from build123d import *

# Parameters (mm, degrees)
SKETCH_1_W          = 100
SKETCH_1_H          = 100
EXTRUDE_1_DEPTH     = 25
SKETCH_2_W          = 100
SKETCH_2_H          = 100
SKETCH_2_W_2        = 8
SKETCH_2_H_2        = 8
CUT_EXTRUDE_1_DEPTH = 20
EXTRUDE_2_REACH     = 145.614
SKETCH_3_R          = 5


with BuildPart() as part:
    # 草图1 → 凸台-拉伸1 (new body)
    with BuildSketch(Plane.XY):
        with Locations((50, 50)):
            Rectangle(SKETCH_1_W, SKETCH_1_H)
    extrude(amount=EXTRUDE_1_DEPTH)

    # 草图2 → 切除-拉伸1 (cut)
    with BuildSketch(Plane.XY.offset(25)):
        with Locations((50, 50)):
            Rectangle(SKETCH_2_W, SKETCH_2_H)
        with Locations((14, 86)):
            Rectangle(SKETCH_2_W_2, SKETCH_2_H_2, mode=Mode.SUBTRACT)
        with Locations((86, 86)):
            Rectangle(SKETCH_2_W_2, SKETCH_2_H_2, mode=Mode.SUBTRACT)
        with Locations((14, 14)):
            Rectangle(SKETCH_2_W_2, SKETCH_2_H_2, mode=Mode.SUBTRACT)
        with Locations((86, 14)):
            Rectangle(SKETCH_2_W_2, SKETCH_2_H_2, mode=Mode.SUBTRACT)
    extrude(amount=-CUT_EXTRUDE_1_DEPTH, mode=Mode.SUBTRACT)

    # 草图3 → 凸台-拉伸2 (add, up to next)
    with BuildSketch(Plane.XY.offset(25), mode=Mode.PRIVATE) as extrude_2_sk1:
        with Locations((50, 50)):
            Circle(SKETCH_3_R)
    extrude_2_tool1 = extrude(extrude_2_sk1.sketch, amount=-EXTRUDE_2_REACH, mode=Mode.PRIVATE) - part.part
    add(extrude_2_tool1.solids().sort_by_distance((50, 50, 25))[0])


solid = part.part
Geometry: final body of the model. Coordinates: model frame, mm. A direction names the side the tool comes from. Give positions to 0.01 mm unless a question says otherwise; leave off trailing zeros. Loops run counter-clockwise (first coordinate to the right, second up) from the corner with the lowest first, then second, coordinate; pieces in that order, holes last. Notation, with made-up numbers: (10, -30) - (61, -30) arc R25 ccw to (61, -12) - close; hole circle Ø4 at (20, 33.5). An arc over 180 degrees is marked (long way). One line per question, with ' | ' between items. Start each with the question number.
(1) Section query B-B on y = 50. Return loops of the section in (x, z), then the cut area to 3 significant figures.
(2) Pull-direction query (X, two-part tool) for faces 1 (the flat face through (82, 14, 15)), 2 (the flat face through (86, 90, 15)), 3 (the flat face through (0, 49, 2)); classes: released by +X, released by -X, zero draft, split by the parting line, or undercut.
(3) Reachability of faces 4 (the flat face through (90, 14, 15)), 5 (the flat face through (10, 86, 15)), 6 (the flat face through (18, 86, 15)), 7 (the flat face through (14, 10, 15)), 8 (the flat face through (86, 18, 15)) from +Z, -Z, +X, -X, +Y, -Y: full face, straight path, thin tool, end or side. Return the list, or none.
(4) Section query A-A on z = 9.5. Return loops of the section in (x, y).
(5) Contact query for flat-ended pins moving along their axis: pin 1 (4 mm diameter, centred on x = 87, z = 11, fed in from +Y); pin 2 (2.5 mm diameter, centred on y = 12.5, z = 20, fed in from -X); pin 3 (6.5 mm diameter, centred on x = 12.5, z = 18.5, fed in from -Y). Output: stop coordinate, or through.
(6) Section query C-C on x = 16. Return loops of the section in (y, z).
(7) Ray query, line 1 (X direction, y = 89, z = 9.5); line 2 (Z direction, x = 60, y = 35). Return the intervals inside material, ascending. Write a range as from..to.
The answers:
1) outline: (0, 0) - (100, 0) - (100, 5) - (55, 5) - (55, 25) - (45, 25) - (45, 5) - (0, 5) - close | area: 700 mm2
2) face 1: undercut | face 2: zero draft | face 3: released by -X
3) face 4: +Z, +X, +Y, -Y | face 5: +Z, -X, +Y, -Y | face 6: +Z, +Y, -Y | face 7: +Z, +X, -X, -Y | face 8: +Z, +X, -X
4) outline: (10, 10) - (18, 10) - (18, 18) - (10, 18) - close; (10, 82) - (18, 82) - (18, 90) - (10, 90) - close; circle Ø10 at (50, 50); (82, 10) - (90, 10) - (90, 18) - (82, 18) - close; (82, 82) - (90, 82) - (90, 90) - (82, 90) - close
5) pin 1: y = 90 | pin 2: x = 10 | pin 3: y = 10
6) outline: (0, 0) - (100, 0) - (100, 5) - (90, 5) - (90, 25) - (82, 25) - (82, 5) - (18, 5) - (18, 25) - (10, 25) - (10, 5) - (0, 5) - close
7) line 1: 10..18, 82..90 | line 2: 0..5
